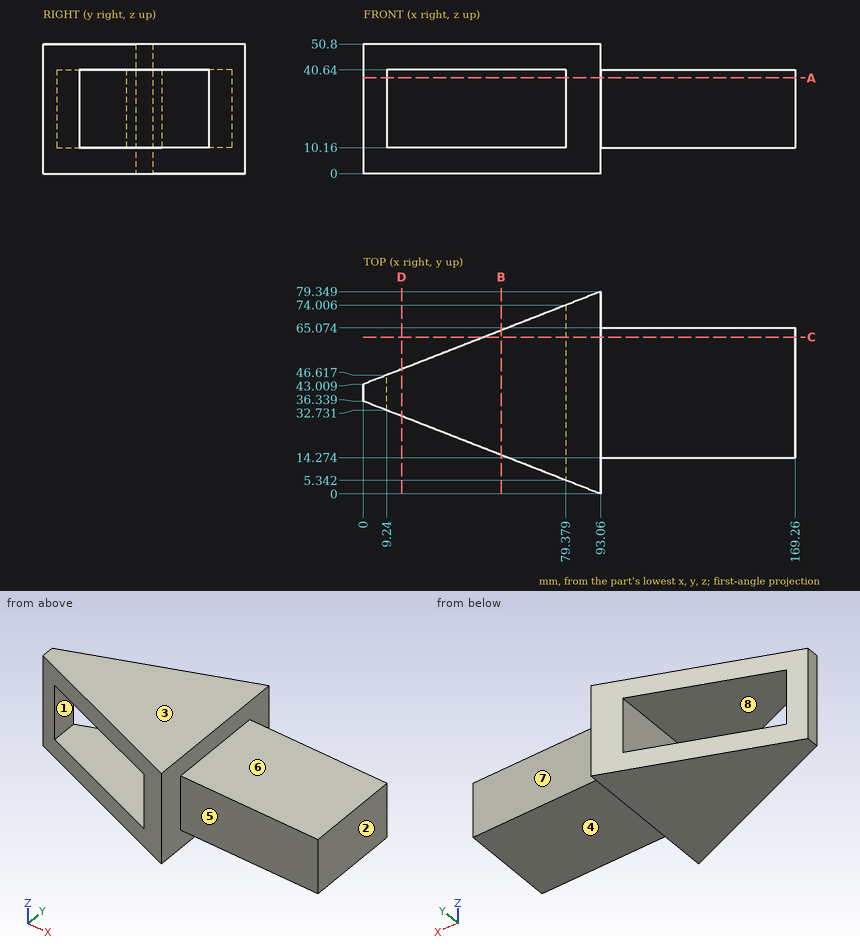
Input: dimensioned drawing with shaded views. Units: mm. Origin: part minimum x, y, z. A direction names the side the tool comes from. Coordinates: 2 decimals unless noted, no trailing zeros. Order: outer loops, then holes, each group sorted by start corner. A loop starts at its lowest first (then second) coordinate and runs counter-clockwise, first axis right, second up. Notation, with made-up numbers: (11.5, 66) -> (18.5, 66) arc R36 cw to (18.5, 105) -> close; hole circle Ø11 at (19, -35.75). An arc over 180 degrees is marked (long way). Answer in a Markdown table with one row per item.
Item 1: Section A-A on z = 37.5. Output: boundary loops of the cut face in (x, y) (1 decimal), plus the area to 3 significant figures.
Return value:
| item | result |
|---|---|
| outline | (0, 36.3) -> (9.2, 32.7) -> (9.2, 46.6) -> (0, 43) -> close; (79.4, 5.3) -> (93.1, 0) -> (93.1, 14.3) -> (169.3, 14.3) -> (169.3, 65.1) -> (93.1, 65.1) -> (93.1, 79.3) -> (79.4, 74) -> close |
| area | 4,980 mm² |
Item 2: Section B-B on x = 54. Output: boundary loops of the cut face in (y, z).
Return value:
| item | result |
|---|---|
| outline | (15.25, 0) -> (64.1, 0) -> (64.1, 10.16) -> (15.25, 10.16) -> close; (15.25, 40.64) -> (64.1, 40.64) -> (64.1, 50.8) -> (15.25, 50.8) -> close |
Item 3: Ray query, L1, parallel to Z at x = 21, y = 46; L2, parallel to X at y = 37, z = 38; L3, parallel to Z at x = 153.5, y = 41.5. Return the intervals inside material, ascending.
Return value:
| item | result |
|---|---|
| L1 | z = 0 to 10.16, 40.64 to 50.8 |
| L2 | x = 0 to 9.24, 79.38 to 169.26 |
| L3 | z = 10.16 to 40.64 |
Item 4: Section D-D on x = 15. Output: boundary loops of the cut face in (y, z).
Return value:
| item | result |
|---|---|
| outline | (30.48, 0) -> (48.87, 0) -> (48.87, 10.16) -> (30.48, 10.16) -> close; (30.48, 40.64) -> (48.87, 40.64) -> (48.87, 50.8) -> (30.48, 50.8) -> close |
Item 5: Contact query for flat-ended pins moving along their axis: P1, Ø3, axis at y = 14, z = 36.5, coming from the -X side; P2, Ø2, axis at x = 143, y = 67.5, coming from the +Z side; P3, Ø1, axis at x = 107.5, y = 65.5, coming from the +Z side; P4, Ø24.5, axis at x = 141.5, z = 24, coming from the +Y side. Output: stop coordinate, or through.
Return value:
| item | result |
|---|---|
| P1 | stops at x = 79.38 |
| P2 | passes through |
| P3 | stops at z = 40.64 |
| P4 | stops at y = 65.07 |
Item 6: Access query for the marked faces 4, 5, 6, 7 and 8. Directions: +Z, -Z, +X, -X, +Y, -Y. A direction counts if a zero-diameter tool reaches every point of the face in a straight line with its end or side. Return the directions, or none.
Return value:
| item | result |
|---|---|
| face 4 | -Z, +X, +Y, -Y |
| face 5 | +Z, -Z, +X, -Y |
| face 6 | +Z, +X, +Y, -Y |
| face 7 | +Z, -Z, +X, +Y |
| face 8 | +Y, -Y |
Item 7: Section C-C on y = 61.5. Output: boundary loops of the cut face in (x, z), plus the area to 3 significant figures.
Return value:
| item | result |
|---|---|
| outline | (47.35, 0) -> (93.06, 0) -> (93.06, 10.16) -> (169.26, 10.16) -> (169.26, 40.64) -> (93.06, 40.64) -> (93.06, 50.8) -> (47.35, 50.8) -> (47.35, 40.64) -> (79.38, 40.64) -> (79.38, 10.16) -> (47.35, 10.16) -> close |
| area | 3,670 mm² |
Item 8: Draft query along X for the marked faces 1, 2 and 3. Return one class per face: released by +X, released by -X, zero draft, split by the parting line, or undercut.
Return value:
| item | result |
|---|---|
| face 1 | undercut |
| face 2 | released by +X |
| face 3 | zero draft |
